Can you work these out from the drawing? Everything is in mm from the part's minimum corner. Round coordinates to 2 decimals unless told otherwise and drop trailing zeros. Loops run counter-clockwise (first coordinate to the right, second up) from the corner with the lowest first, then second, coordinate; pieces in that order, holes last. Notation, with made-up numbers: (57.5, 61.5) -> (82.5, 61.5) arc R18 cw to (82.5, 94.5) -> close; hole circle Ø9 at (-32.5, -22.75). An arc over 180 degrees is marked (long way). Answer as a JSON object with one key per item and string values.
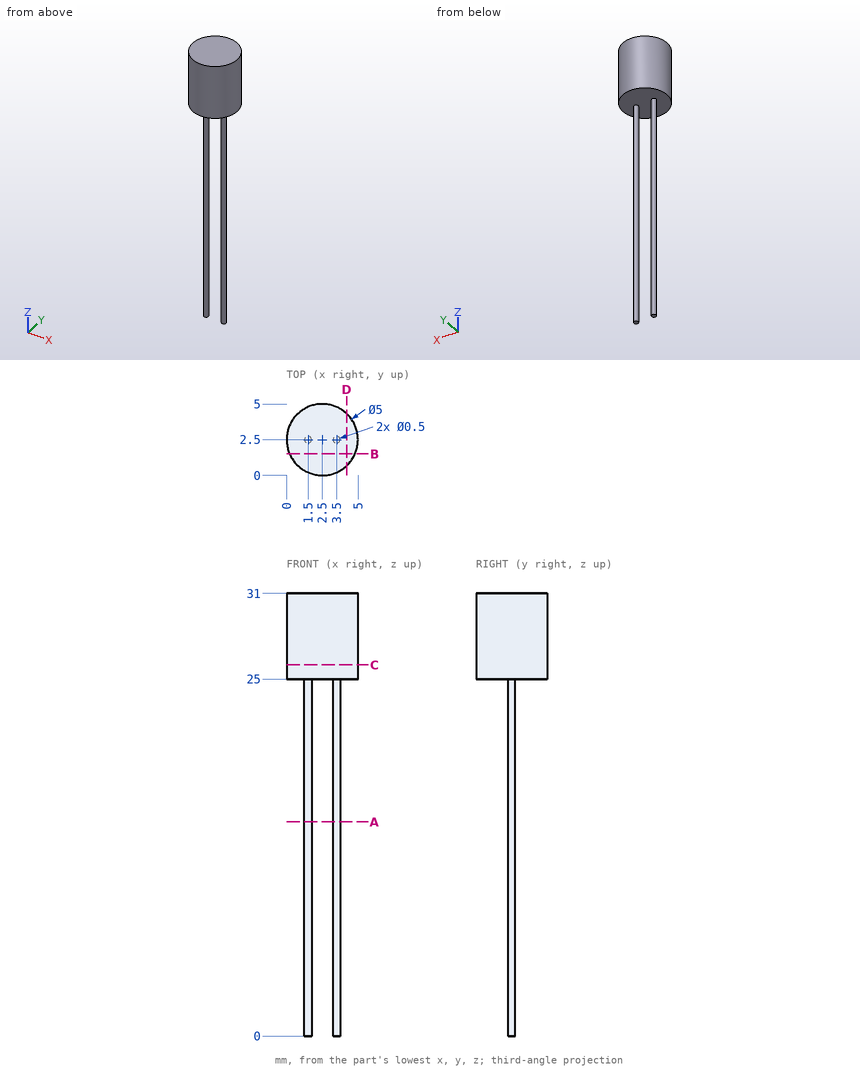
Q1. I want a section at C-C, the plane z = 26. Write out the boundary of the cut face in (x, y), then the cut area to 3 significant figures.
Determined:
{"outline": "circle Ø5 at (2.5, 2.5)", "area": "19.6 mm²"}
Q2. If I drill on L1, parallel to Z at x = 4.7, y = 1.9; L2, parallel to Y at x = 3.7, z = 3; L3, parallel to X at y = 4, z = 27, over which ranges is the centre line in solid material (lowest first)? Write a range as [from, to].
Determined:
{"L1": "[25, 31]", "L2": "[2.35, 2.65]", "L3": "[0.5, 4.5]"}
Q3. I want a section at D-D, the plane x = 4.2. Write out the boundary of the cut face in (y, z), then the cut area to 3 significant figures.
Determined:
{"outline": "(0.67, 25) -> (4.33, 25) -> (4.33, 31) -> (0.67, 31) -> close", "area": "22.0 mm²"}
Q4. I want a section at B-B, the plane y = 1.5. Write out the boundary of the cut face in (x, z).
Determined:
{"outline": "(0.21, 25) -> (4.79, 25) -> (4.79, 31) -> (0.21, 31) -> close"}
Q5. I want a section at A-A, the plane z = 15. Write out the boundary of the cut face in (x, y).
Determined:
{"outline": "circle Ø0.5 at (1.5, 2.5); circle Ø0.5 at (3.5, 2.5)"}
